from build123d import *

# Parameters (mm, degrees)
F1_DEPTH = 25
F2_W     = 25
F2_H     = 36.3502395384
F3_DEPTH = 5
F4_R     = 3
F5_DEPTH = 12


with BuildPart() as f1:
    # F0 (on Right) → F1 (new body)
    with BuildSketch(Plane.YZ):
        Polygon((0, 89.97), (0, 0), (36.3502395384, 0), align=None)
    extrude(amount=F1_DEPTH)

    # F2 (on face) → F3 (join)
    with BuildSketch(Plane(origin=(0, 0, 0), x_dir=(1, 0, 0), z_dir=(0, 0, -1))):
        with Locations((12.5, -18.1751197692)):
            Rectangle(F2_W, F2_H)
    extrude(amount=F3_DEPTH)

    # F4 (on face) → F5 (cut)
    with BuildSketch(Plane(origin=(0, 31.2492067951, 12.6254990818), x_dir=(-1, 0, 0), z_dir=(0, 0.9271838546, 0.3746065934))):
        with Locations((-12.5, 34.900845996)):
            Circle(F4_R)
        with Locations((-12.5, 59.8668195307)):
            Circle(F4_R)
        with Locations((-12.5, 9.9348724613)):
            Circle(F4_R)
    extrude(amount=-F5_DEPTH, mode=Mode.SUBTRACT)


solid = f1.part
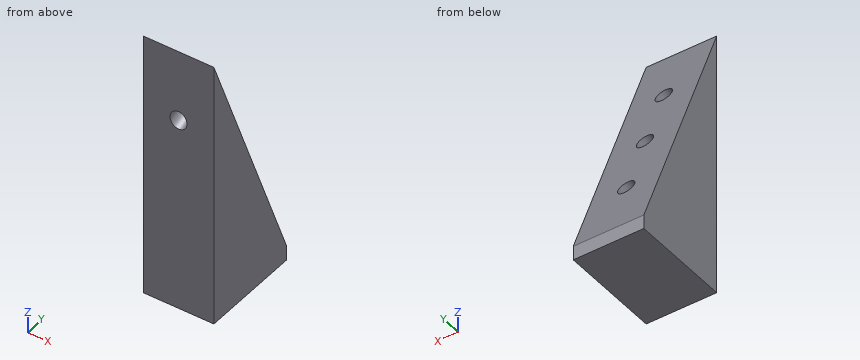
The listing builds one solid part. Answer for the finished solid, in the listing's coordinates (mm). Give positions to 0.01 mm unless a question says otherwise; leave off trailing zeros. Write each loop counter-clockwise with the first axis right and the second up, starting at its lowest first coordinate (ties: lowest second). Pieces come first, ordered by that corner, then holes. Notation, with made-up numbers: (81, 54.5) - (111, 54.5) arc R23 cw to (111, 77.5) - close; hole circle Ø7 at (-22.75, 32.25). An arc over 180 degrees is marked (long way). Use a Markdown table: item, result.
1. Each of these flat-tipped pins is pushed along its axis until it touches: P1, Ø1.5, axis at x = 22, y = 19.5, coming from the +Z side; P2, Ø8, axis at x = 6, y = 12, coming from the +Z side. Where does it stop, or does it pass through?
Values follow:
| item | result |
|---|---|
| P1 | stops at z = 43.56 |
| P2 | stops at z = 70.17 |
2. Section B-B on z = 5.5 is taken. Write down the section's boundary in (x, y), plus the area to 3 significant figures.
Values follow:
| item | result |
|---|---|
| outline | (0, 0) - (25, 0) - (25, 34.13) - (0, 34.13) - close |
| area | 853 mm² |
3. Find the intervals of material crossed by probe 1 along X at (y, z) = (21.5, 18); probe 2 along X at (y, z) = (21, 18); probe 3 along Z at (x, y) = (11.5, 2), in increasing order. Write a range as from..to.
Values follow:
| item | result |
|---|---|
| probe 1 | x = 0..9.8, 15.2..25 |
| probe 2 | x = 0..9.71, 15.29..25 |
| probe 3 | z = -5..62.33, 68.43..85.02 |
4. Section A-A on x = 16.5 is taken. Write down the section's boundary in (y, z).
Values follow:
| item | result |
|---|---|
| outline | (0, -5) - (36.35, -5) - (36.35, 0) - (0, 89.97) - close |
